Could you check a few things on this model? Use its own coordinates, in mm. A direction names the side the tool comes from. Round coordinates to 2 decimals unless told otherwise and drop trailing zeros. Write each loop counter-clockwise with the first axis right and the second up, starting at its lowest first coordinate (ties: lowest second). Pieces come first, ordered by that corner, then holes. Notation, with made-up numbers: (69, 35) -> (112, 35) arc R25 ccw to (112, 74) -> close; hole circle Ø6 at (-22.75, 27). An arc over 180 degrees is marked (long way). Answer as CSV lines item,"result". Start each with the question number.
Q1. Imagine slicing it at B-B on y = 18. Please give me the cut outline in (x, z).
Q2. Will these pins go through, and if not, where does the flat tip stop? pin 1 Ø12 at (x, z) = (5, 17) entering from +Y; pin 2 Ø1.5 at (y, z) = (59.5, 34.5) entering from +X; pin 3 Ø9 at (x, y) = (6.5, 72) entering from -Z.
Q3. Imagine slicing it at A-A on x = 16. Please give me the cut outline in (y, z), and give its area (3 significant figures).
Q4. Imagine slicing it at C-C on z = -11. Please give me the cut outline in (x, y), and give its area (3 significant figures).
Q5. If I drill on line 1 (Y direction, x = 16, z = 50.85); line 2 (Z direction, x = 5.5, y = 24.5); line 3 (Z direction, x = -17.15, y = 71), over which ranges is the centre line in solid material (lowest first)? Write a range as [from, to].
Q6. For faces 5 (the flat face through (-20, 33, 1)), 6 (the flat face through (2, 39, -48.5)), 7 (the flat face through (1, 71, 50.5)), 8 (the flat face through (1, 71, -50.5)), which set-ups out of +Z, -Z, +X, -X, +Y, -Y let a thin tool reach every point of the face, with its end or its side?
Q7. Imagine slicing it at D-D on y = 71. Please give me the cut outline in (x, z).
Q8. If we mould it in two halves opening along Y, with no side actions, what happens to faces 1 (the flat face through (20, 1, 0)), 2 (the cylindrical face through (-17.014, 72.537, -0.202)), 3 (the cylindrical face through (16.336, 44.487, -50.472)), 4 (the flat face through (2, 4, 1))? For each: pulls with the +Y half, pulls with the -Y half, needs draft (parallel to the pull), parting line crosses it, or undercut.
from build123d import *

# Parameters (mm, degrees)
SKETCH1_W               = 40
SKETCH1_H               = 105
BOSS_EXTRUDE3_DEPTH     = 75
SKETCH4_W               = 97
SKETCH4_H               = 71
CUT_EXTRUDE2_DEPTH      = 36
SKETCH5_W               = 40
SKETCH5_H               = 8
CUT_EXTRUDE3_DEPTH      = 2
SKETCH6_W               = 40
SKETCH6_H               = 8
CUT_EXTRUDE4_DEPTH      = 2
SKETCH7_W               = 101
SKETCH7_H               = 8
CUT_EXTRUDE5_DEPTH      = 2
SKETCH8_R               = 1.55
CUT_EXTRUDE6_DEPTH      = 102
CUT_EXTRUDE6_DEPTH_BACK = 5
SKETCH10_R              = 1.55
CUT_EXTRUDE8_DEPTH      = 2


with BuildPart() as part:
    # Sketch1 → Boss-Extrude3 (new body)
    with BuildSketch(Plane(origin=(0, 0, 0), x_dir=(1, 0, 0), z_dir=(0, 1, 0))):
        Rectangle(SKETCH1_W, SKETCH1_H)
    extrude(amount=BOSS_EXTRUDE3_DEPTH)

    # Sketch4 → Cut-Extrude2 (cut)
    with BuildSketch(Plane(origin=(20, 0, 0), x_dir=(0, 0, -1), z_dir=(1, 0, 0))):
        with Locations((0, 39.5)):
            Rectangle(SKETCH4_W, SKETCH4_H)
    extrude(amount=-CUT_EXTRUDE2_DEPTH, mode=Mode.SUBTRACT)

    # Sketch5 → Cut-Extrude3 (cut)
    with BuildSketch(Plane.XY.offset(52.5)):
        with Locations((0, 71)):
            Rectangle(SKETCH5_W, SKETCH5_H)
    extrude(amount=-CUT_EXTRUDE3_DEPTH, mode=Mode.SUBTRACT)

    # Sketch6 → Cut-Extrude4 (cut)
    with BuildSketch(Plane(origin=(0, 0, -52.5), x_dir=(-1, 0, 0), z_dir=(0, 0, -1))):
        with Locations((0, 71)):
            Rectangle(SKETCH6_W, SKETCH6_H)
    extrude(amount=-CUT_EXTRUDE4_DEPTH, mode=Mode.SUBTRACT)

    # Sketch7 → Cut-Extrude5 (cut)
    with BuildSketch(Plane.ZY.offset(20)):
        with Locations((0, 71)):
            Rectangle(SKETCH7_W, SKETCH7_H)
    extrude(amount=-CUT_EXTRUDE5_DEPTH, mode=Mode.SUBTRACT)

    # Sketch8 → Cut-Extrude6 (cut, two sides)
    with BuildSketch(Plane(origin=(0, 0, 48.5), x_dir=(-1, 0, 0), z_dir=(0, 0, -1))) as cut_extrude6_sk:
        with Locations((-16, 18)):
            Circle(SKETCH8_R)
        with Locations((-16, 46)):
            Circle(SKETCH8_R)
    extrude(amount=CUT_EXTRUDE6_DEPTH, mode=Mode.SUBTRACT)
    extrude(cut_extrude6_sk.sketch, amount=-CUT_EXTRUDE6_DEPTH_BACK, mode=Mode.SUBTRACT)

    # Sketch10 → Cut-Extrude8 (cut)
    with BuildSketch(Plane.ZY.offset(18)):
        with Locations((0, 71)):
            Circle(SKETCH10_R)
    extrude(amount=-CUT_EXTRUDE8_DEPTH, mode=Mode.SUBTRACT)


solid = part.part
Checks:
1,outline,"(-20, -52.5) -> (14.45, -52.5) -> (14.45, -48.5) -> (-16, -48.5) -> (-16, 48.5) -> (14.45, 48.5) -> (14.45, 52.5) -> (-20, 52.5) -> close; (17.55, -52.5) -> (20, -52.5) -> (20, -48.5) -> (17.55, -48.5) -> close; (17.55, 48.5) -> (20, 48.5) -> (20, 52.5) -> (17.55, 52.5) -> close"
2,pin 1,"y = 4"
2,pin 2,"x = -16"
2,pin 3,"z = -50.5"
3,outline,"(0, -52.5) -> (16.45, -52.5) -> (16.45, -48.5) -> (4, -48.5) -> (4, 48.5) -> (16.45, 48.5) -> (16.45, 52.5) -> (0, 52.5) -> close; (19.55, -52.5) -> (44.45, -52.5) -> (44.45, -48.5) -> (19.55, -48.5) -> close; (19.55, 48.5) -> (44.45, 48.5) -> (44.45, 52.5) -> (19.55, 52.5) -> close; (47.55, -52.5) -> (67, -52.5) -> (67, -50.5) -> (75, -50.5) -> (75, -48.5) -> (47.55, -48.5) -> close; (47.55, 48.5) -> (75, 48.5) -> (75, 50.5) -> (67, 50.5) -> (67, 52.5) -> (47.55, 52.5) -> close"
3,area,"906 mm^2"
4,outline,"(-20, 0) -> (20, 0) -> (20, 4) -> (-16, 4) -> (-16, 75) -> (-18, 75) -> (-18, 67) -> (-20, 67) -> close"
4,area,"428 mm^2"
5,line 1,"[0, 16.45], [19.55, 44.45], [47.55, 67]"
5,line 2,"[-52.5, -48.5], [48.5, 52.5]"
5,line 3,"[-50.5, -1.55], [1.55, 50.5]"
6,face 5,"+Z, -Z, -X, +Y, -Y"
6,face 6,"+X, +Y"
6,face 7,"+Z, +X, -X, +Y"
6,face 8,"-Z, +X, -X, +Y"
7,outline,"(-18, -50.5) -> (20, -50.5) -> (20, -48.5) -> (-16, -48.5) -> (-16, -1.55) -> (-18, -1.55) -> close; (-18, 1.55) -> (-16, 1.55) -> (-16, 48.5) -> (20, 48.5) -> (20, 50.5) -> (-18, 50.5) -> close"
8,face 1,"needs draft"
8,face 2,"undercut"
8,face 3,"undercut"
8,face 4,"pulls with the +Y half"
